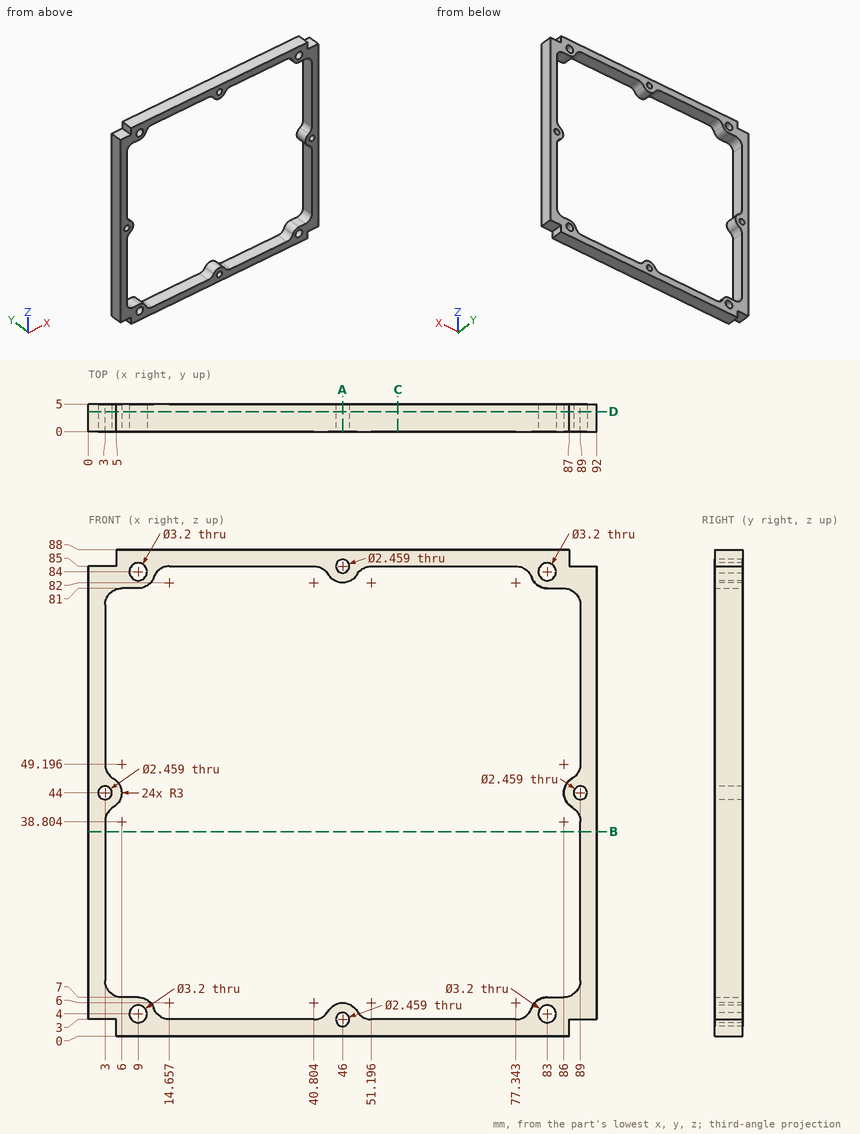
Drawing for the job (mm, zero at the part's lowest x, y, z). Coordinates: 2 decimals unless noted, no trailing zeros. Order: outer loops, then holes, each group sorted by start corner. A loop starts at its lowest first (then second) coordinate and runs counter-clockwise, first axis right, second up. Notation, with made-up numbers: (0, 20.25) - (56, 20.25) arc R26 ccw to (56, 55.25) - close; hole circle Ø3 at (67.5, -25). An arc over 180 degrees is marked (long way). Use a Markdown table: item, result. Add a question column.
(1) Flat gauge pins, fed straight in: pin 1 (0.9 mm diameter, centred on y = 2.5, z = 1.5, fed in from +X); pin 2 (2.5 mm diameter, centred on x = 1.5, y = 3.5, fed in from +Z); pin 3 (1.5 mm diameter, centred on y = 2.5, z = 1, fed in from -X). Where does each tip first touch, or does it go through?
(2) Saw through at C-C (x = 56). Give the cut face in (y, z).
(3) Drill centre lines: line 1 along Z through (x, y) = (46, 2.7); line 2 along Z through (x, y) = (83, 1.5); line 3 along X through (y, z) = (2.7, 44). Where is each one in solid material? Low to high. Write a range as [from, to].
(4) Saw through at D-D (y = 3.6). Count the separate pieces of the cut face and the enclosed holes in it, then the cut area to 3 significant figures.
(5) Saw through at B-B (z = 37). Give the cut face in (x, y).
(6) Saw through at A-A (x = 46). Give the cut face in (y, z).
Solved:
| question | item | result |
|---|---|---|
| 1 | pin 1 | stops at x = 87 |
| 1 | pin 2 | stops at z = 85 |
| 1 | pin 3 | stops at x = 5 |
| 2 | outline | (0, 0) - (5, 0) - (5, 3) - (0, 3) - close; (0, 85) - (5, 85) - (5, 88) - (0, 88) - close |
| 3 | line 1 | z = [0, 1.77], [4.23, 6], [82, 83.77], [86.23, 88] |
| 3 | line 2 | z = [0, 2.4], [5.6, 7], [81, 82.4], [85.6, 88] |
| 3 | line 3 | x = [0, 1.77], [4.23, 6], [86, 87.77], [90.23, 92] |
| 4 | separate pieces | 1 |
| 4 | enclosed holes | 9 |
| 4 | area | 1,140 mm² |
| 5 | outline | (0, 0) - (3, 0) - (3, 5) - (0, 5) - close; (89, 0) - (92, 0) - (92, 5) - (89, 5) - close |
| 6 | outline | (0, 0) - (5, 0) - (5, 1.77) - (0, 1.77) - close; (0, 4.23) - (5, 4.23) - (5, 6) - (0, 6) - close; (0, 82) - (5, 82) - (5, 83.77) - (0, 83.77) - close; (0, 86.23) - (5, 86.23) - (5, 88) - (0, 88) - close |
